Part model, mm, in its own coordinate system. Face numbers are marked on the shaded views. A direction names the side the tool comes from. Round coordinates to 2 decimals unless told otherwise and drop trailing zeros. Loops run counter-clockwise (first coordinate to the right, second up) from the corner with the lowest first, then second, coordinate; pieces in that order, holes last. Notation, with made-up numbers: (53.25, 7.5) -> (99.25, 7.5) arc R11 cw to (99.25, 28.5) -> close; hole circle Ø5 at (-39.75, -40). An arc over 180 degrees is marked (long way). Use a Markdown table: item, result. Add a question column.
Item 1: Probe line 1 (Z direction, x = -1313, y = -3); line 2 (Z direction, x = -2276, y = 0); line 3 (X direction, y = 0, z = -58). List the from-to ranges inside material, lowest first. Write a range as [from, to].
Item 2: Cut at A-A, the plane x = -1574. List the corners of the cut face in (y, z), plus the area to 3 significant figures.
Item 3: Which spindle directions (+Z, -Z, +X, -X, +Y, -Y) get a long thin tool onto all of the face, cutting with end or side? Do the marked faces 1 and 2. Say none if no direction does.
Item 4: Flat gauge pins, fed straight in: pin 1 (4 mm diameter, centred on x = -1590, y = 45.5, fed in from -Z); pin 2 (2 mm diameter, centred on x = -1755.5, y = 44.5, fed in from +Z); pin 3 (3 mm diameter, centred on x = -2212, z = 3, fed in from +Y); pin 4 (1.7 mm diameter, centred on x = -1673.91, z = 0, fed in from +Y). Where does each tip first touch, or does it go through?
```python
from build123d import *

# Parameters (mm, degrees)
SKETCH2_R          = 1.4224
CUT_EXTRUDE1_DEPTH = 20
CIRPATTERN1_COUNT  = 8


with BuildPart() as part:
    # Sketch1 → Revolve1 (revolve)
    with BuildSketch(Plane.XY):
        Polygon((-1238.910735908, 59.93638), (-2246.556635908, 59.93638), (-2246.556635908, 57.15), (-2373.556635908, 57.15), (-2373.556635908, 54.36362), (-2119.556635908, 54.36362), (-2119.556635908, 57.15), (-1238.910735908, 57.15), align=None)
    revolve(axis=Axis((-2246.556635908, 0, 0), (1, 0, 0)))

    # Sketch2 → Cut-Extrude1 (cut)
    with BuildSketch(Plane(origin=(0, 0, -59.93638), x_dir=(-1, 0, 0), z_dir=(0, 0, -1))):
        with Locations((1673.910735908, 0)):
            Circle(SKETCH2_R)
    cut_extrude1 = extrude(amount=-CUT_EXTRUDE1_DEPTH, mode=Mode.SUBTRACT)

    # CirPattern1: Cut-Extrude1 ×8 about axis
    cirpattern1_axis = Axis((-1238.910735908, 0, 0), (-1, 0, 0))
    for i in range(1, CIRPATTERN1_COUNT):
        add(cut_extrude1.rotate(cirpattern1_axis, i * 360 / CIRPATTERN1_COUNT), mode=Mode.SUBTRACT)


solid = part.part
```
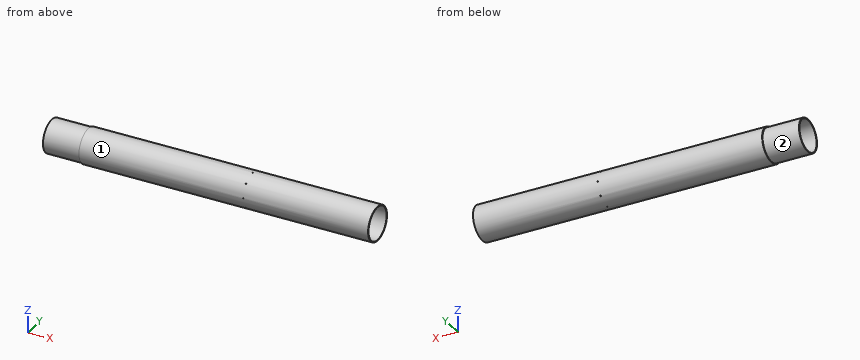
A:
| question | item | result |
|---|---|---|
| 1 | line 1 | z = [-59.86, -57.07], [57.07, 59.86] |
| 1 | line 2 | z = [-57.15, -54.36], [54.36, 57.15] |
| 1 | line 3 | x = [-2246.56, -1675.33], [-1672.49, -1238.91] |
| 2 | outline | circle Ø119.87 at (0, 0); hole circle Ø114.3 at (0, 0) |
| 2 | area | 1,020 mm^2 |
| 3 | face 1 | +X, -X |
| 3 | face 2 | -X |
| 4 | pin 1 | stops at z = -41.23 |
| 4 | pin 2 | stops at z = 41.23 |
| 4 | pin 3 | stops at y = 59.92 |
| 4 | pin 4 | passes through |
